from build123d import *

# Parameters (mm, degrees)
BOSS_EXTRUDE1_DEPTH     = 12.7
BOSS_EXTRUDE1_2_DEPTH   = 12.7
BOSS_EXTRUDE1_3_DEPTH   = 12.7
BOSS_EXTRUDE1_4_DEPTH   = 12.7
BOSS_EXTRUDE2_DEPTH     = 6.35
CUT_EXTRUDE2_DEPTH      = 471.19349296362236
CUT_EXTRUDE2_DEPTH_BACK = 471.19349296362236


with BuildPart() as part:
    # Sketch2 → Boss-Extrude1 (new body)
    with BuildSketch(Plane(origin=(0, 0, 0), x_dir=(1, 0, 0), z_dir=(0, 1, 0))):
        with BuildLine():
            Line((173.83852694696787, 6.353879523850983), (173.83852694696787, 107.95387952385097))
            ThreePointArc((173.83852694696787, 107.95387952385097), (175.69702705818847, 112.4426365219853), (180.18464742311625, 114.30387952385061))
            Line((180.18464742311625, 114.30387952385061), (180.18464742311627, 120.65387952385097))
            Line((180.18464742311627, 120.65387952385097), (154.78464742311627, 120.65387952385103))
            Line((154.78464742311627, 120.65387952385103), (154.78464742311627, 114.30387952385061))
            ThreePointArc((154.78464742311627, 114.30387952385061), (159.27728359825178, 112.44537975999239), (161.1385269469677, 107.95387952385097))
            Line((161.1385269469677, 107.95387952385097), (161.1385269469677, 6.353879523850983))
            ThreePointArc((161.1385269469677, 6.353879523850983), (159.28002683574687, 1.8651225257164699), (154.79240647081883, 0.00387952385118295))
            Line((154.79240647081883, 0.00387952385118295), (154.79240647081883, -6.34612047614902))
            Line((154.79240647081883, -6.34612047614902), (180.19240647081884, -6.34612047614902))
            Line((180.19240647081884, -6.34612047614902), (180.19240647081887, 0.00387952385118295))
            ThreePointArc((180.19240647081887, 0.00387952385118295), (175.69977029568358, 1.8623792877096292), (173.83852694696787, 6.353879523850983))
        make_face()
    extrude(amount=BOSS_EXTRUDE1_DEPTH)



with BuildPart() as body_2:
    # Sketch2 → Boss-Extrude1 2 (new body)
    with BuildSketch(Plane(origin=(0, 0, 0), x_dir=(1, 0, 0), z_dir=(0, 1, 0))):
        with BuildLine():
            Line((290.5044221112303, -6.346119624362247), (290.50442211122953, 107.95388037563158))
            ThreePointArc((290.50442211122953, 107.95388037563158), (292.3629222224477, 112.44263737377035), (296.8505425873776, 114.30388037563806))
            Line((296.8505425873776, 114.30388037563806), (296.8505425873776, 120.65388037564047))
            Line((296.8505425873776, 120.65388037564047), (271.45054258737764, 120.65388037564018))
            Line((271.45054258737764, 120.65388037564018), (271.4505425873777, 114.30388037563777))
            ThreePointArc((271.4505425873777, 114.30388037563777), (275.94317876251387, 112.44538061177975), (277.80442211123, 107.95388037563791))
            Line((277.80442211123, 107.95388037563791), (277.80442211123005, 15.745570535197672))
            Line((277.80442211123005, 15.745570535197672), (212.3933170880388, 120.65388037563798))
            Line((212.3933170880388, 120.65388037563798), (188.7491541871168, 120.65388037563798))
            Line((188.7491541871168, 120.65388037563798), (188.7491541871168, 114.30388037563738))
            ThreePointArc((188.7491541871168, 114.30388037563738), (197.0586174651338, 109.87545758746259), (203.35223987593548, 102.87199949093673))
            Line((203.35223987593548, 102.87199949093673), (203.35223987593548, 6.353880375637708))
            ThreePointArc((203.35223987593548, 6.353880375637708), (201.49271132298225, 1.8640946501521807), (197.00321001616626, 0.00387952385096785))
            Line((197.00321001616626, 0.00387952385096785), (197.00321001616626, -6.34612047614902))
            Line((197.00321001616626, -6.34612047614902), (222.4032100161663, -6.34612058725173))
            Line((222.4032100161663, -6.34612058725173), (222.4027250756679, 0.00387939423115991))
            ThreePointArc((222.4027250756679, 0.00387939423115991), (217.91228324219506, 1.8635802308402507), (216.0522403203464, 6.353880375637722))
            Line((216.0522403203464, 6.353880375637722), (216.0522403203464, 82.50335442487922))
            Line((216.0522403203464, 82.50335442487922), (271.45054277255036, -6.346119624362282))
            Line((271.45054277255036, -6.346119624362282), (290.5044221112303, -6.346119624362247))
        make_face()
    extrude(amount=BOSS_EXTRUDE1_2_DEPTH)


with BuildPart() as body_3:
    # Sketch2 → Boss-Extrude1 3 (new body)
    with BuildSketch(Plane(origin=(0, 0, 0), x_dir=(1, 0, 0), z_dir=(0, 1, 0))):
        with BuildLine():
            ThreePointArc((379.8796721750226, 11.977744632292787), (390.1923529413957, 3.169883174382882), (403.37970421101926, 0.00388024601806133))
            Line((403.37970421101926, 0.00388024601806133), (403.37970421101926, -6.346119753981942))
            Line((403.37970421101926, -6.346119753981942), (365.27970421101924, -6.346119753981938))
            Line((365.27970421101924, -6.346119753981938), (365.2797042110193, 0.00388024601805613))
            ThreePointArc((365.2797042110193, 0.00388024601805613), (369.3036929855622, 2.4697837385241583), (368.9334095604214, 7.174680748774959))
            Line((368.9334095604214, 7.174680748774959), (330.73082744761575, 59.756024084156806))
            Line((330.73082744761575, 59.756024084156806), (324.38179758784645, 53.88870851238104))
            Line((324.38179758784645, 53.88870851238104), (324.38179758784645, 6.353880042329715))
            ThreePointArc((324.38179758784645, 6.353880042329715), (326.24184092866363, 1.8635806636905663), (330.7322823430498, 0.00388024601804399))
            Line((330.7322823430498, 0.00388024601804399), (330.73276728366636, -6.346119735464957))
            Line((330.73276728366636, -6.346119735464957), (305.3327672836663, -6.346119624362247))
            Line((305.3327672836663, -6.346119624362247), (305.3327672836663, 0.00388037563774091))
            ThreePointArc((305.3327672836663, 0.00388037563774091), (309.8222685904823, 1.8640955019389631), (311.6817971434355, 6.3538812274244805))
            Line((311.6817971434355, 6.3538812274244805), (311.6817971434355, 107.95388156073302))
            ThreePointArc((311.6817971434355, 107.95388156073302), (309.82175422158684, 112.44418170553047), (305.331312388114, 114.30388254213955))
            Line((305.331312388114, 114.30388254213955), (305.33082744761555, 120.65388252362244))
            Line((305.33082744761555, 120.65388252362244), (330.7308274476156, 120.65388241251989))
            Line((330.7308274476156, 120.65388241251989), (330.73082744761564, 114.3038824125199))
            ThreePointArc((330.73082744761564, 114.3038824125199), (326.241326559762, 112.4436677052449), (324.38179758784645, 107.95388274582793))
            Line((324.38179758784645, 107.95388274582793), (324.38179758784645, 61.00818587469014))
            Line((324.38179758784645, 61.00818587469014), (370.01136074815463, 103.17573782782141))
            ThreePointArc((370.01136074815463, 103.17573782782141), (371.6316997254356, 110.22586005871784), (365.6567975878465, 114.30388241251993))
            Line((365.6567975878465, 114.30388241251993), (365.6567975878465, 120.65388241251989))
            Line((365.6567975878465, 120.65388241251989), (397.4067975878465, 120.65388241251989))
            Line((397.4067975878465, 120.65388241251989), (397.4067975878465, 114.3038824125199))
            ThreePointArc((397.4067975878465, 114.3038824125199), (390.28312138184594, 112.95972058249937), (384.1390825743689, 109.11208223600183))
            Line((384.1390825743689, 109.11208223600183), (339.36773990380823, 67.7376357737456))
            Line((339.36773990380823, 67.7376357737456), (379.8796721750226, 11.977744632292787))
        make_face()
    extrude(amount=BOSS_EXTRUDE1_3_DEPTH)


with BuildPart() as body_4:
    # Sketch2 → Boss-Extrude1 4 (new body)
    with BuildSketch(Plane(origin=(0, 0, 0), x_dir=(1, 0, 0), z_dir=(0, 1, 0))):
        with BuildLine():
            Line((0, -6.35), (127, -6.35))
            Line((127, -6.35), (133.835466699924, -6.35))
            Line((133.835466699924, -6.35), (142.41022736904142, 24.2201812141727))
            Line((142.41022736904142, 24.2201812141727), (137.42037994397373, 24.2201812141727))
            ThreePointArc((137.42037994397373, 24.2201812141727), (127.07789830370176, 9.03099759553653), (109.65993293339864, 3.1750000000000025))
            Line((109.65993293339864, 3.1750000000000025), (38.100000000000165, 3.1750000000000007))
            ThreePointArc((38.100000000000165, 3.1750000000000007), (24.629615818396296, 8.754615818396267), (19.050000000000022, 22.225000000000133))
            Line((19.050000000000022, 22.225000000000133), (19.049999999999997, 222.25))
            ThreePointArc((19.049999999999997, 222.25), (21.531156391441193, 228.66169963567893), (27.681998366018952, 231.7330466139162))
            Line((27.681998366018952, 231.7330466139162), (27.68199836601896, 241.2580466139162))
            Line((27.68199836601896, 241.2580466139162), (-10.418001633981042, 241.2580466139162))
            Line((-10.418001633981042, 241.2580466139162), (-10.418001633981042, 231.7330466139162))
            ThreePointArc((-10.418001633981042, 231.7330466139162), (-3.1133003643210593, 229.2938436085588), (0, 222.25))
            Line((0, 222.25), (0, 16.260176542443787))
            ThreePointArc((0, 16.260176542443787), (-3.8325594762586483, 7.0075594762586455), (-13.085176542443792, 3.1750000000000007))
            Line((-13.085176542443792, 3.1750000000000007), (-13.085176542443786, -6.35))
            Line((-13.085176542443786, -6.35), (0, -6.35))
        make_face()
    extrude(amount=BOSS_EXTRUDE1_4_DEPTH)


with BuildPart() as part_1:
    add(part.part)

    add(body_2.part)  # Boss-Extrude2 merges body 2

    add(body_3.part)  # Boss-Extrude2 merges body 3

    add(body_4.part)  # Boss-Extrude2 merges body 4
    # Sketch4 → Boss-Extrude2 (add)
    with BuildSketch(Plane(origin=(0, 0, 0), x_dir=(1, 0, 0), z_dir=(0, 1, 0))):
        Polygon((136.68158195989426, 3.7967857367812146), (376.38878950850017, 4.555259431461488), (376.38878950850017, 10.146785736781245), (136.68158195989426, 10.146785736781215), align=None)
    extrude(amount=BOSS_EXTRUDE2_DEPTH)

    # Sketch6 → Cut-Extrude2 (cut, two sides: drawn at the far end of the back side and taken through both)
    with BuildSketch(Plane(origin=(0, 12.7, 0), x_dir=(1, 0, 0), z_dir=(0, 1, 0)).offset(-CUT_EXTRUDE2_DEPTH_BACK)):
        with BuildLine():
            Line((324.6925686344705, 4.391683942646109), (369.79590978466945, 4.534398457384592))
            ThreePointArc((369.79590978466945, 4.534398457384592), (369.57267914306925, 5.922493261126043), (368.9334095604214, 7.174680748774945))
            Line((368.9334095604214, 7.174680748774945), (366.77404888893807, 10.146785736781244))
            Line((366.77404888893807, 10.146785736781244), (324.38179758784645, 10.146785736781238))
            Line((324.38179758784645, 10.146785736781238), (324.38179758784645, 6.353880042329715))
            ThreePointArc((324.38179758784645, 6.353880042329715), (324.4599715437991, 5.360553286293043), (324.6925686344705, 4.391683942646109))
        make_face()
        with BuildLine():
            Line((216.4851967942631, 4.049297720927505), (264.8734590646552, 4.202406275479168))
            Line((264.8734590646552, 4.202406275479168), (261.16709462286485, 10.14678573678123))
            Line((261.16709462286485, 10.14678573678123), (216.0522403203464, 10.146785736781224))
            Line((216.0522403203464, 10.146785736781224), (216.0522403203464, 6.353880375637722))
            ThreePointArc((216.0522403203464, 6.353880375637722), (216.16141789373137, 5.181430727271779), (216.4851967942631, 4.049297720927505))
        make_face()
    extrude(amount=CUT_EXTRUDE2_DEPTH + CUT_EXTRUDE2_DEPTH_BACK, mode=Mode.SUBTRACT)


solid = part_1.part
Here's how the part is built. I have some questions about the finished solid (model axes, mm). A direction names the side the tool comes from. Coordinates: 2 decimals unless noted, no trailing zeros. Write each loop counter-clockwise with the first axis right and the second up, starting at its lowest first coordinate (ties: lowest second). Pieces come first, ordered by that corner, then holes.
1) If I drill on line 1 (X direction, y = 12, z = -117); line 2 (Z direction, x = 105, y = 2.25) (3 decimals); line 3 (X direction, y = 3.25, z = -143), over which ranges is the centre line in solid material (lowest first)?
Filled in:
line 1: x = 0 to 19.05, 154.78 to 180.18, 188.75 to 214.67, 271.45 to 296.85, 305.33 to 330.73, 365.66 to 397.41
line 2: z = -3.175 to 6.35
line 3: x = 0 to 19.05
2) Which directions (+Z, -Z, +X, -X, +Y, -Y) give clear straight access to the entire face, cutting with the end or side of a thin tool? Please do faces 1 (the face through (24.779, 6.261, -8.607)), 2 (the face through (390.02, 6.26, -3.26)), 3 (the face through (127.3, 6.3, -9.2)), 4 (the face through (27.682, 6, -236)).
Filled in:
face 1: +Y, -Y
face 2: +X, +Y, -Y
face 3: -Z, +Y, -Y
face 4: -Z, +X, +Y, -Y
3) I'm going to push flat-ended pins straight in: pin 1 (4 mm diameter, centred on x = 240.5, y = 6.5, fed in from -Z); pin 2 (4 mm diameter, centred on x = 139, y = 7, fed in from -Z); pin 3 (4 mm diameter, centred on x = 280, y = 6.5, fed in from +Z). Where does each tip first touch, or does it pass through?
Filled in:
pin 1: stops at z = -78.78
pin 2: stops at z = -24.22
pin 3: stops at z = 6.35
4) If we section it at A-A (z = -34.5): List the corners of the cut face in (x, y) for me, plus the area to 3 significant figures.
Filled in:
outline: (0, 0) - (19.05, 0) - (19.05, 12.7) - (0, 12.7) - close; (161.14, 0) - (173.84, 0) - (173.84, 12.7) - (161.14, 12.7) - close; (203.35, 0) - (216.05, 0) - (216.05, 12.7) - (203.35, 12.7) - close; (245.98, 0) - (266.11, 0) - (266.11, 12.7) - (245.98, 12.7) - close; (277.8, 0) - (290.5, 0) - (290.5, 12.7) - (277.8, 12.7) - close; (311.68, 0) - (324.38, 0) - (324.38, 12.7) - (311.68, 12.7) - close; (349.08, 0) - (363.52, 0) - (363.52, 12.7) - (349.08, 12.7) - close
area: 1,330 mm2
5) If we section it at B-B (x = 353.5): List the corners of the cut face in (y, z) for me.
Filled in:
outline: (0, -87.92) - (12.7, -87.92) - (12.7, -80.8) - (0, -80.8) - close; (0, -48.29) - (12.7, -48.29) - (12.7, -28.42) - (0, -28.42) - close
6) Thinking about a two-plate mould opening in Z: for faces 5 (the face through (216.052, 6, -44)), 6 (the face through (344, 12.7, -48)), 7 (the face through (168, 6, -120.654)), which applies, +Z half, -Z half, draft (parallel to the pull), parting line (faces both ways), or undercut?
Filled in:
face 5: undercut
face 6: draft
face 7: -Z half
7) If we section it at C-C (z = -160): List the corners of the cut face in (x, y) for me, plus the area to 3 significant figures.
Filled in:
outline: (0, 0) - (19.05, 0) - (19.05, 12.7) - (0, 12.7) - close
area: 242 mm2
8) If we section it at D-D (x = 63): List the corners of the cut face in (y, z) for me (3 decimals), plus the area to 3 significant figures.
Filled in:
outline: (0, -3.175) - (12.7, -3.175) - (12.7, 6.35) - (0, 6.35) - close
area: 121 mm2
